from build123d import *

# Parameters (mm, degrees)
EXTRUDE_1_DEPTH     = 15
SKETCH_2_OUTSIDE_W  = 37.634
SKETCH_2_OUTSIDE_H  = 33.922
SKETCH_2_OUTSIDE_R  = 6
CUT_EXTRUDE_1_DEPTH = 10


with BuildPart() as part:
    # Эскиз1 → Бобышка-Вытянуть1 (new body)
    with BuildSketch(Plane(origin=(0, 0, 0), x_dir=(1, 0, 0), z_dir=(0, 1, 0))):
        Polygon((13.856406461, 0), (6.92820323, 12), (-6.92820323, 12), (-13.856406461, 0), (-6.92820323, -12), (6.92820323, -12), align=None)
    extrude(amount=EXTRUDE_1_DEPTH)

    # Эскиз2 outside → Вырез-Вытянуть1 (cut)
    with BuildSketch(Plane(origin=(0, 15, 0), x_dir=(1, 0, 0), z_dir=(0, 1, 0))):
        Rectangle(SKETCH_2_OUTSIDE_W, SKETCH_2_OUTSIDE_H)
        with Locations(Location((0, 0, 0), (0, 0, 270))):
            Circle(SKETCH_2_OUTSIDE_R, mode=Mode.SUBTRACT)
    extrude(amount=-CUT_EXTRUDE_1_DEPTH, mode=Mode.SUBTRACT)


solid = part.part
Here's how the part is built. I have some questions about the finished solid (model axes, mm). A direction names the side the tool comes from. Coordinates: 2 decimals unless noted, no trailing zeros. Order: outer loops, then holes, each group sorted by start corner. A loop starts at its lowest first (then second) coordinate and runs counter-clockwise, first axis right, second up. Notation, with made-up numbers: (87, 38.5) -> (118, 38.5) arc R22 ccw to (118, 63.5) -> close; hole circle Ø1 at (-16.5, 55). An arc over 180 degrees is marked (long way). Answer in a Markdown table with one row per item.
(1) I want a section at D-D on y = 8.5. List the corners of the cut face in (x, z) for me.
Answer key:
| item | result |
|---|---|
| outline | circle Ø12 at (0, 0) |
(2) I want a section at B-B on y = 2.5. List the corners of the cut face in (x, z) for me.
Answer key:
| item | result |
|---|---|
| outline | (-13.86, 0) -> (-6.93, -12) -> (6.93, -12) -> (13.86, 0) -> (6.93, 12) -> (-6.93, 12) -> close |
(3) I want a section at C-C on z = 1.5. List the corners of the cut face in (x, y) for me.
Answer key:
| item | result |
|---|---|
| outline | (-12.99, 0) -> (12.99, 0) -> (12.99, 5) -> (5.81, 5) -> (5.81, 15) -> (-5.81, 15) -> (-5.81, 5) -> (-12.99, 5) -> close |
(4) Will these pins go through, and if not, where does the flat tip stop? pin 1 Ø1 at (y, z) = (6, 4.5) entering from -X; pin 2 Ø3 at (x, z) = (-7, -5) entering from +Y; pin 3 Ø3 at (x, y) = (-1.5, 11) entering from -Z; pin 4 Ø5 at (x, z) = (-7.5, 2) entering from -Y.
Answer key:
| item | result |
|---|---|
| pin 1 | x = -4.47 |
| pin 2 | y = 5 |
| pin 3 | z = -6 |
| pin 4 | y = 0 |
(5) On a 3-axis mill with a long thin cutter (end or side, diameter ignored), from which of +Z, -Z, +X, -X, +Y, -Y can I reach the whole of each face in a straight line? I mean faces 1 (the face through (0, 15, 0)), 2 (the face through (3, 5, -6)). Say none if no direction works.
Answer key:
| item | result |
|---|---|
| face 1 | +Z, -Z, +X, -X, +Y |
| face 2 | +Y |
(6) I want a section at A-A on x = 0. List the corners of the cut face in (y, z) for me.
Answer key:
| item | result |
|---|---|
| outline | (0, -12) -> (5, -12) -> (5, -6) -> (15, -6) -> (15, 6) -> (5, 6) -> (5, 12) -> (0, 12) -> close |
(7) Please list where these lines run through material, in increasing order: probe 1 along Y at (x, z) = (-2.75, -8.5); probe 2 along X at (y, z) = (11.25, 0); probe 3 along Z at (x, y) = (-3, 8.75).
Answer key:
| item | result |
|---|---|
| probe 1 | 0 to 5 |
| probe 2 | -6 to 6 |
| probe 3 | -5.2 to 5.2 |
